For this review, take the finished solid that the model builds, in its own axes (mm). Face numbers are marked on the shaded views. Round coordinates to 2 decimals unless told otherwise and drop trailing zeros. Loops run counter-clockwise (first coordinate to the right, second up) from the corner with the lowest first, then second, coordinate; pieces in that order, holes last.
1) Take a section at A-A (x = 0). State the section outline as (y, z) points, then the cut area to 3 significant figures.
2) Wall thickness on L1, parallel to Z at x = 0, y = -73; L2, parallel to Z at x = 0, y = -38.5; L3, parallel to Y at x = 5, z = -5: over which ranges is each line inside the solid? List them lowest first.
3) Take a section at B-B (y = -19). State the section outline as (x, z) points, then the cut area to 3 significant figures.
4) Insertion check: pin 1 (3 mm diameter, centred on y = -45.5, z = 5, fed in from +X); pin 2 (10.5 mm diameter, centred on x = 0, z = 0, fed in from +Y); pin 3 (1 mm diameter, centred on y = -93, z = 1.5, fed in from -X); pin 4 (2 mm diameter, centred on x = 1.5, z = -1, fed in from +Y). Each pin has a flat end and moves straight along its axis. Give the tip position at first contact, or say it passes through.
5) Take a section at C-C (z = -4.75). State the section outline as (x, y) points, then the cut area to 3 significant figures.
6) Take a section at D-D (y = -106). State the section outline as (x, z) points, then the cut area to 3 significant figures.
7) Mouldability with a two-part tool opening along Z and no side actions: class the marked faces 1, 2 and 3 as pulls with the +Z half, pulls with the -Z half, needs draft (parallel to the pull), parting line crosses it, or undercut.
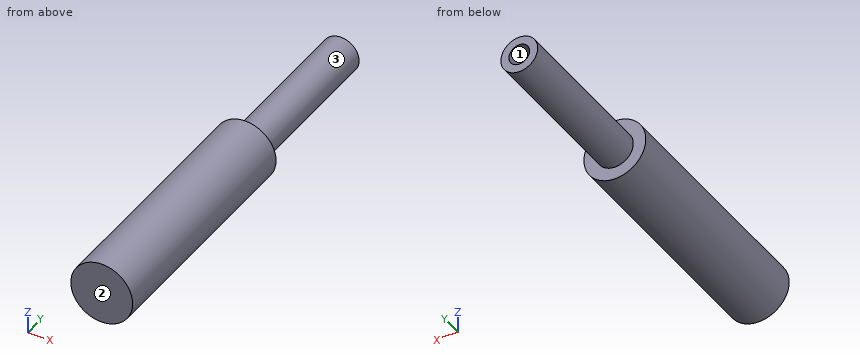
```python
from build123d import *

# Parameters (mm, degrees)
F0_W     = 5.799088
F0_H     = 50.8
F2_R     = 3.25962
F3_DEPTH = 82.296


with BuildPart() as f1:
    # F0 (on Top) → F1 (revolve)
    with BuildSketch(Plane.XY):
        with Locations((2.899544, -25.4)):
            Rectangle(F0_W, F0_H)
        Polygon((5.799088, -50.8), (0, -50.8), (0, -127), (9.742463, -127), (9.742463, -50.8), align=None)
    revolve(axis=Axis((0, -63.5, 0), (0, -1, 0)))


with BuildPart() as f3:
    # F2 (on Front) → F3 (new body)
    with BuildSketch(Plane.XZ):
        Circle(F2_R)
    extrude(amount=F3_DEPTH)


with BuildPart() as f1_1:
    add(f1.part)

    # F4: cut F3
    add(f3.part, mode=Mode.SUBTRACT)


solid = f1_1.part
```
Response:
1. outline: (-127, -9.74) - (-50.8, -9.74) - (-50.8, -5.8) - (0, -5.8) - (0, -3.26) - (-82.3, -3.26) - (-82.3, 3.26) - (0, 3.26) - (0, 5.8) - (-50.8, 5.8) - (-50.8, 9.74) - (-127, 9.74) - close
1. area: 1,540 mm2
2. L1: z = -9.74 to -3.26, 3.26 to 9.74
2. L2: z = -5.8 to -3.26, 3.26 to 5.8
2. L3: y = -127 to -50.8
3. outline: circle Ø11.6 at (0, 0); hole circle Ø6.52 at (0, 0)
3. area: 72.3 mm2
4. pin 1: stops at x = 4.62
4. pin 2: stops at y = 0
4. pin 3: stops at x = -9.69
4. pin 4: stops at y = -82.3
5. outline: (-8.51, -127) - (8.51, -127) - (8.51, -50.8) - (3.33, -50.8) - (3.33, 0) - (-3.33, 0) - (-3.33, -50.8) - (-8.51, -50.8) - close
5. area: 1,630 mm2
6. outline: circle Ø19.48 at (0, 0)
6. area: 298 mm2
7. face 1: undercut
7. face 2: needs draft
7. face 3: parting line crosses it
